Geometry check sheet. Reference: drawing and pictorial views, mm from the part's lowest x, y, z. Coordinates: 2 decimals unless noted, no trailing zeros. Order: outer loops, then holes, each group sorted by start corner. A loop starts at its lowest first (then second) coordinate and runs counter-clockwise, first axis right, second up. Notation, with made-up numbers: M -15.5,56.25 L 5.5,56.25 A17 ccw 5.5,82.25 Z; hole C -15.5,-1.75 d11. An arc over 180 degrees is marked long. Return JSON: item names as keys, results as strings.
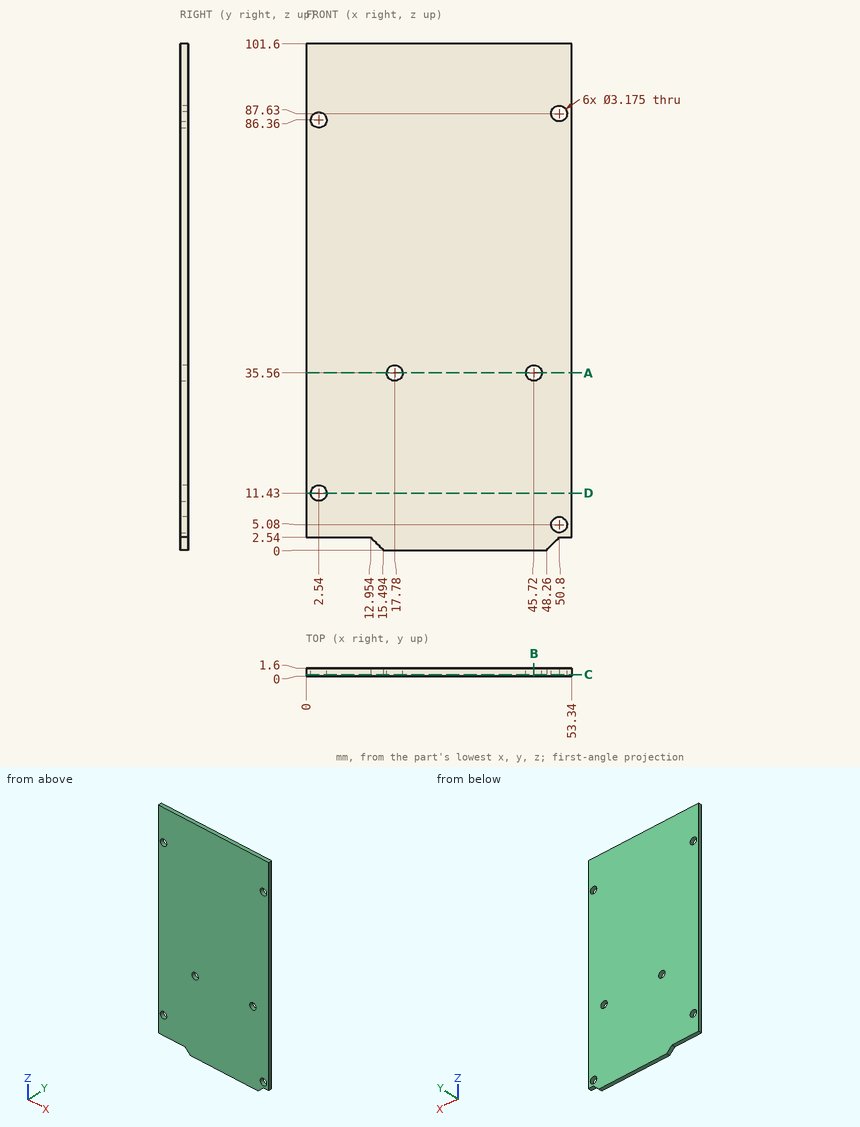
Q1. Cross-section at D-D, the plane z = 11.43. Record the boundary of the cut face in (x, y), and give its area (3 significant figures).
Values:
{"outline": "M 0,0 L 0.95,0 L 0.95,1.6 L 0,1.6 Z; M 4.13,0 L 53.34,0 L 53.34,1.6 L 4.13,1.6 Z", "area": "80.3 mm^2"}
Q2. Cross-section at A-A, the plane z = 35.56. Record the boundary of the cut face in (x, y).
Values:
{"outline": "M 0,0 L 16.19,0 L 16.19,1.6 L 0,1.6 Z; M 19.37,0 L 44.13,0 L 44.13,1.6 L 19.37,1.6 Z; M 47.31,0 L 53.34,0 L 53.34,1.6 L 47.31,1.6 Z"}
Q3. Cross-section at B-B, the plane x = 45.72. Record the boundary of the cut face in (y, z).
Values:
{"outline": "M 0,0 L 1.6,0 L 1.6,33.97 L 0,33.97 Z; M 0,37.15 L 1.6,37.15 L 1.6,101.6 L 0,101.6 Z"}
Q4. Go/stop test with a flat-tipped pin: pin 1 (0.5 mm diameter, centred on x = 5.5, y = 1, fed in from -Z). Record where the tip stops, or that it passes through.
Values:
{"pin 1": "z = 2.54"}
Q5. Material ranges on line 1 along X through (y, z) = (0.4, 35.56); line 2 along X through (y, z) = (0.8, 86.36); line 3 along Z through (x, y) = (17.78, 0.5), recorded low to high.
Values:
{"line 1": "0 to 16.19, 19.37 to 44.13, 47.31 to 53.34", "line 2": "0 to 0.95, 4.13 to 49.85, 51.75 to 53.34", "line 3": "0 to 33.97, 37.15 to 101.6"}
Q6. Cross-section at C-C, the plane y = 0.3. Record the boundary of the cut face in (x, z) (1 decimal), and give its area (3 significant figures).
Values:
{"outline": "M 0,2.5 L 13,2.5 L 15.5,0 L 48.3,0 L 50.8,2.5 L 53.3,2.5 L 53.3,101.6 L 0,101.6 Z; hole C 2.5,11.4 d3.2; hole C 2.5,86.4 d3.2; hole C 17.8,35.6 d3.2; hole C 45.7,35.6 d3.2; hole C 50.8,5.1 d3.2; hole C 50.8,87.6 d3.2", "area": "5,330 mm^2"}
